Read the model definition and answer for the solid it produces. Units are mm, in the model's axes. Face numbers are marked on the shaded views. A direction names the side the tool comes from. Round coordinates to 2 decimals unless told otherwise and drop trailing zeros. Order: outer loops, then holes, each group sorted by start corner. A loop starts at its lowest first (then second) coordinate and runs counter-clockwise, first axis right, second up. Notation, with made-up numbers: (82, -27) - (140, -27) arc R8 ccw to (140, -14) - close; hole circle Ø10 at (47.5, 76.5). An arc over 180 degrees is marked (long way). One line per question, with ' | ' between items. Start each with the question number.
1) Straight lines are drawn through the part: line 1 (Z direction, x = 12.5, y = 14); line 2 (Y direction, x = 87, z = -93). For each, find the intervals that lie inside material, in ascending order. Write a range as from..to.
2) The mould has two halves that part along Y. Classify the marked faces 1, 2, 3 and 4: pulls with the +Y half, pulls with the -Y half, needs draft (parallel to the pull), parting line crosses it, or undercut.
3) The part is cut by section A-A, the plane z = 54.5. Give the vertices of the cut face in (x, y), plus the area to 3 significant figures.
4) The part is cut by section C-C, the plane x = 89. Give the vertices of the cut face in (y, z), plus the area to 3 significant figures.
5) For the marked faces 5 and 6, determine the directions among +Z, -Z, +X, -X, +Y, -Y from which every point of the face is accessible in a straight line to the end or side of a thin tool.
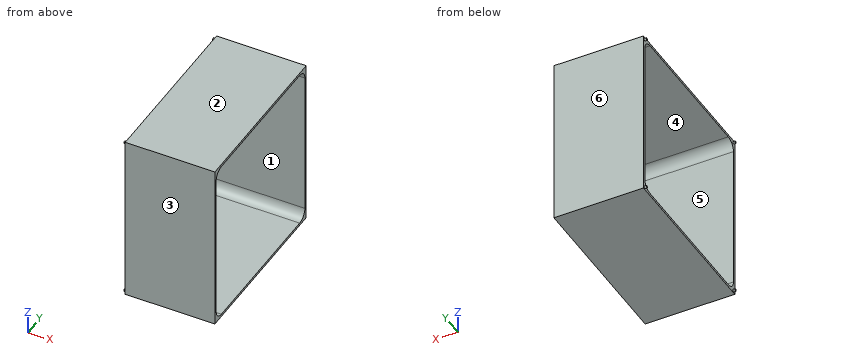
from build123d import *

# Parameters (mm, degrees)
SKETCH1_W               = 210
SKETCH1_H               = 210
BOSS_EXTRUDE1_DEPTH     = 110
SKETCH2_W               = 204
SKETCH2_H               = 204
CUT_EXTRUDE1_DEPTH      = 110
FILLET1_R               = 12
SKETCH3_R               = 1.5
BOSS_EXTRUDE2_DEPTH     = 2.5
MIRROR2_COPY_1_SKETCH_R = 1.5
MIRROR2_COPY_1_DEPTH    = 2.5


with BuildPart() as part:
    # Sketch1 → Boss-Extrude1 (new body)
    with BuildSketch(Plane(origin=(0, 0, 0), x_dir=(0, 0, -1), z_dir=(1, 0, 0))):
        Rectangle(SKETCH1_W, SKETCH1_H)
    extrude(amount=BOSS_EXTRUDE1_DEPTH)

    # Sketch2 → Cut-Extrude1 (cut)
    with BuildSketch(Plane(origin=(110, 0, 0), x_dir=(0, 0, -1), z_dir=(1, 0, 0))):
        Rectangle(SKETCH2_W, SKETCH2_H)
    extrude(amount=-CUT_EXTRUDE1_DEPTH, mode=Mode.SUBTRACT)

    # Fillet1
    fillet1_edges = [part.edges().sort_by_distance(p)[0] for p in [
        (55, -102, -102),
        (55, -102, 102),
        (55, 102, 102),
        (55, 102, -102),
    ]]
    fillet(fillet1_edges, radius=FILLET1_R)

    # Sketch3 → Boss-Extrude2 (add)
    with BuildSketch(Plane.ZY):
        with Locations((-102, 102)):
            Circle(SKETCH3_R)
    boss_extrude2 = extrude(amount=BOSS_EXTRUDE2_DEPTH)

    # Mirror1: Boss-Extrude2 across plane
    add(boss_extrude2.mirror(Plane.XY))

    # Mirror2: Boss-Extrude2 across plane
    add(boss_extrude2.mirror(Plane.ZX))

    # Mirror2 copy 1 sketch → Mirror2 copy 1 (add)
    with BuildSketch(Plane(origin=(0, 0, 0), x_dir=(0, 0, -1), z_dir=(-1, 0, 0))):
        with Locations((-102, 102)):
            Circle(MIRROR2_COPY_1_SKETCH_R)
    extrude(amount=MIRROR2_COPY_1_DEPTH)


solid = part.part
Values:
1) line 1: z = -105..-102, 102..105 | line 2: y = -105..-101.62, 101.62..105
2) face 1: undercut | face 2: needs draft | face 3: pulls with the -Y half | face 4: undercut
3) outline: (0, -105) - (110, -105) - (110, -102) - (0, -102) - close; (0, 102) - (110, 102) - (110, 105) - (0, 105) - close | area: 660 mm^2
4) outline: (-105, -105) - (105, -105) - (105, 105) - (-105, 105) - close; hole (-102, -90) arc R12 ccw to (-90, -102) - (90, -102) arc R12 ccw to (102, -90) - (102, 90) arc R12 ccw to (90, 102) - (-90, 102) arc R12 ccw to (-102, 90) - close | area: 2,610 mm^2
5) face 5: +X, -X | face 6: +Z, -Z, +X, -X, +Y
